Input: part model. Units: mm. Frame: model coordinates. Give positions to 0.01 mm unless a question says otherwise; leave off trailing zeros. Loops run counter-clockwise (first coordinate to the right, second up) from the corner with the lowest first, then second, coordinate; pieces in that order, holes last. Notation, with made-up numbers: (-24.5, -6.75) - (-19.5, -6.75) arc R27 ccw to (-19.5, 16.25) - close; hole circle Ø8 at (48, -34.5). An arc over 180 degrees is marked (long way). One line per item, written item: value.
from build123d import *

# Parameters (mm, degrees)
SKETCH_1_R          = 0.75
SKETCH_1_R_2        = 0.3
EXTRUDE_1_DEPTH     = 1
FILLET_1_R          = 0.1
EXTRUDE_2_DEPTH     = 40
SKETCH_3_R          = 2.953544
CUT_EXTRUDE_1_DEPTH = 20
SKETCH_4_W          = 0.74162
SKETCH_4_H          = 0.3
EXTRUDE_3_DEPTH     = 5.5
SKETCH_6_R          = 0.15
CUT_EXTRUDE_2_DEPTH = 5.5
FILLET_2_R          = 0.3


with BuildPart() as part:
    # 草图1 → 凸台-拉伸1 (new body)
    with BuildSketch(Plane.XY):
        with Locations((0.75, 0)):
            Circle(SKETCH_1_R)
        with Locations((0.75, 0)):
            Circle(SKETCH_1_R_2, mode=Mode.SUBTRACT)
    extrude(amount=EXTRUDE_1_DEPTH)

    # 圆角1
    fillet_1_edges = [part.edges().sort_by_distance(p)[0] for p in [
        (0, 0, 1),
        (0, 0, 0),
    ]]
    fillet(fillet_1_edges, radius=FILLET_1_R)

    # 草图2 → 凸台-拉伸2 (add)
    with BuildSketch(Plane(origin=(0, -0.3, 0), x_dir=(-1, 0, 0), z_dir=(0, 1, 0))):
        with BuildLine():
            ThreePointArc((-0.35, 0.5), (-0.652986, 0.888057), (-1.102941, 0.688235))
            Line((-1.102941, 0.688235), (-0.397059, 0.311765))
            ThreePointArc((-0.397059, 0.311765), (-0.361943, 0.402986), (-0.35, 0.5))
        make_face()
        with BuildLine():
            Line((-0.397059, 0.311765), (-1.102941, 0.688235))
            ThreePointArc((-1.102941, 0.688235), (-0.938235, 0.147059), (-0.397059, 0.311765))
        make_face()
    extrude(amount=-EXTRUDE_2_DEPTH)

    # 草图3 → 切除-拉伸1 (cut)
    with BuildSketch(Plane.XZ.offset(40.3)):
        with Locations((0.75, 0.5)):
            Circle(SKETCH_3_R)
    extrude(amount=-CUT_EXTRUDE_1_DEPTH, mode=Mode.SUBTRACT)

    # 草图4 → 凸台-拉伸3 (add)
    with BuildSketch(Plane.XZ.offset(20.3)):
        with Locations((0.75, 0.5)):
            Rectangle(SKETCH_4_W, SKETCH_4_H)
    extrude(amount=EXTRUDE_3_DEPTH)

    # 草图6 → 切除-拉伸2 (cut)
    with BuildSketch(Plane(origin=(0, 0, 0.35), x_dir=(-1, 0, 0), z_dir=(0, 0, -1))):
        with Locations((-0.737636, -25.336312)):
            Circle(SKETCH_6_R)
    extrude(amount=-CUT_EXTRUDE_2_DEPTH, mode=Mode.SUBTRACT)

    # 圆角2
    fillet_2_edges = [part.edges().sort_by_distance(p)[0] for p in [
        (1.12081, -25.8, 0.5),
        (0.37919, -25.8, 0.5),
    ]]
    fillet(fillet_2_edges, radius=FILLET_2_R)


solid = part.part
Item 1: Section A-A, the plane y = 0. Output: boundary loops of the cut face in (x, z).
Verdict:
outline: (0, 0.1) arc R0.1 ccw to (0.1, 0) - (0.45, 0) - (0.45, 1) - (0.1, 1) arc R0.1 ccw to (0, 0.9) - close; (1.05, 0) - (1.4, 0) arc R0.1 ccw to (1.5, 0.1) - (1.5, 0.9) arc R0.1 ccw to (1.4, 1) - (1.05, 1) - close
Item 2: Material intervals for L1, parallel to Y at x = 0.75, z = 0.2; L2, parallel to Y at x = 0.75, z = 0.5; L3, parallel to X at y = -2, z = 0.45, sorted ascending.
Verdict:
L1: y = -20.3 to -0.3, 0.3 to 0.75
L2: y = -25.8 to -25.49, -25.19 to -0.3, 0.3 to 0.75
L3: x = 0.35 to 1.15
Item 3: Section B-B, the plane y = -6.5. Output: boundary loops of the cut face in (x, z).
Verdict:
outline: (0.35, 0.5) arc R0.4 ccw to (0.4, 0.31) arc R0.4 ccw (long way) to start
